Autodesk Inventor part; units mm, degrees
ref_plane "YZ Plane" through (0, 0, 0) normal (1, 0, 0) x (0, 1, 0)
ref_plane "XZ Plane" through (0, 0, 0) normal (0, 1, 0) x (-1, 0, 0)
ref_plane "XY Plane" through (0, 0, 0) normal (0, 0, 1) x (1, 0, 0)
sketch "Sketch1" plane through (0, 0, 0) normal (0, 1, 0) x (-1, 0, 0)
  circle A0 centre (2.4819, 9.1831) radius 0.635
  point P0 (0, 0)
  dimension "d0" = 1.27
extrude "Extrusion1" add sketch "Sketch1" along normal blind 304.8
sketch "Sketch2" plane through (-2.4819, 304.8, 9.1831) normal (0, 1, 0) x (1, 0, 0)
  line L0 (-1.0816, -1.7196) -> (0.8833, -1.7196)
  line L1 (0.8833, -1.7196) -> (0.8833, 1.4308)
  line L2 (0.8833, 1.4308) -> (-1.0816, 1.4308)
  line L3 (-1.0816, 1.4308) -> (-1.0816, -1.7196)
  point P0 (2.4819, 9.1831)
extrude "Extrusion2" add sketch "Sketch2" along normal blind 12.7
sketch "Sketch3" plane through (-2.4819, 317.5, 9.1831) normal (0, 1, 0) x (1, 0, 0)
  line L0 (-0.7645, -1.2984) -> (0.6263, -1.2984)
  line L1 (0.6263, -1.2984) -> (0.6263, -1.1087)
  line L2 (0.6263, -1.1087) -> (-0.7645, -1.1087)
  line L3 (-0.7645, -1.1087) -> (-0.7645, -1.2984)
  line L4 (-0.7645, 0.6885) -> (0.5541, 0.6885)
  line L5 (0.5541, 0.6885) -> (0.5541, 0.8962)
  line L6 (0.5541, 0.8962) -> (-0.7645, 0.8962)
  line L7 (-0.7645, 0.8962) -> (-0.7645, 0.6885)
  point P0 (2.4819, 9.1831)
extrude "Extrusion3" add sketch "Sketch3" along normal blind 6.35
properties part number "plug"
Work out the finished part from the listing and answer in its coordinate system (mm). Round coordinates to 2 decimals unless told otherwise and drop trailing zeros. Write each loop counter-clockwise with the first axis right and the second up, starting at its lowest first coordinate (ties: lowest second). Pieces come first, ordered by that corner, then holes. Notation, with made-up numbers: (82.5, -27.5) - (98.5, -27.5) arc R15 ccw to (98.5, -3.5) - close; hole circle Ø11 at (-9, -3). An arc over 180 degrees is marked (long way). Answer in a Markdown table with one row per item. Add a question column.
1. A cutting plane is placed at A-A, the plane x = -2.7. Determine the outline of the cut face in (y, z).
2. Find the intervals of material crossed by line 1 along Y through (x, z) = (-2.3, 9.05); line 2 along Y through (x, z) = (-2, 8); line 3 along Z through (x, y) = (-2.7, 248), in increasing order. Write a range as from..to.
3. A cutting plane is placed at B-B, the plane y = 221. Determine the outline of the cut face in (x, z) (3 decimals).
4. Given pin 1 (1.1 mm diameter, centred on x = -2.5, y = 322, fed in from +Z); pin 2 (1 mm diameter, centred on x = -2.5, y = 147.5, fed in from -Z), each flat-ended and moving along its own axis, determine where each tip first touches the part or whether it passes through.
Worked out:
| question | item | result |
|---|---|---|
| 1 | outline | (0, 8.59) - (304.8, 8.59) - (304.8, 7.75) - (317.5, 7.75) - (317.5, 8.29) - (323.85, 8.29) - (323.85, 8.49) - (317.5, 8.49) - (317.5, 10.29) - (323.85, 10.29) - (323.85, 10.48) - (317.5, 10.48) - (317.5, 10.9) - (304.8, 10.9) - (304.8, 9.78) - (0, 9.78) - close |
| 2 | line 1 | 0..317.5 |
| 2 | line 2 | 304.8..317.5 |
| 2 | line 3 | 8.59..9.78 |
| 3 | outline | circle Ø1.27 at (-2.482, 9.183) |
| 4 | pin 1 | z = 10.48 |
| 4 | pin 2 | z = 8.55 |
